from build123d import *

# Parameters (mm, degrees)
SKETCH1_W           = 22.225
SKETCH1_H           = 12.7
BOSS_EXTRUDE1_DEPTH = 50.8
SKETCH2_R           = 1.905
CUT_EXTRUDE1_DEPTH  = 57.884801353
CUT_EXTRUDE2_DEPTH  = 56.811406764
FILLET1_R           = 1.5875
SKETCH6_R           = 2.286
CUT_EXTRUDE3_DEPTH  = 57.884801482


with BuildPart() as part:
    # Sketch1 → Boss-Extrude1 (new body)
    with BuildSketch(Plane(origin=(0, 0, 0), x_dir=(1, 0, 0), z_dir=(0, 1, 0))):
        with Locations((11.1125, 6.35)):
            Rectangle(SKETCH1_W, SKETCH1_H)
    extrude(amount=BOSS_EXTRUDE1_DEPTH)

    # Sketch2 → Cut-Extrude1 (cut, through all)
    with BuildSketch(Plane(origin=(0, 0, -12.7), x_dir=(-1, 0, 0), z_dir=(0, 0, -1))):
        with Locations((-17.4625, 44.45)):
            Circle(SKETCH2_R)
        with Locations((-17.4625, 6.35)):
            Circle(SKETCH2_R)
        with Locations((-4.7625, 44.45)):
            Circle(SKETCH2_R)
        with Locations((-4.7625, 6.35)):
            Circle(SKETCH2_R)
    extrude(amount=-CUT_EXTRUDE1_DEPTH, mode=Mode.SUBTRACT)

    # Sketch3 → Cut-Extrude2 (cut, through all)
    with BuildSketch(Plane(origin=(0, 0, -6.35), x_dir=(-1, 0, 0), z_dir=(0, 0, -1))):
        with BuildLine():
            Line((0, 10.541), (0, 2.159))
            Line((0, 2.159), (-0.79375, 2.159))
            ThreePointArc((-0.79375, 2.159), (-1.786060968, 2.860879553), (-2.286, 3.96875))
            Line((-2.286, 3.96875), (-2.286, 8.73125))
            ThreePointArc((-2.286, 8.73125), (-1.786060968, 9.839120447), (-0.79375, 10.541))
            Line((-0.79375, 10.541), (0, 10.541))
        make_face()
    extrude(amount=-CUT_EXTRUDE2_DEPTH, mode=Mode.SUBTRACT)

    # Sketch5 → Cut-Revolve2 (revolve, cut)
    with BuildSketch(Plane(origin=(0, 0, -6.35), x_dir=(-1, 0, 0), z_dir=(0, 0, -1))):
        with BuildLine():
            Line((0, 6.35), (-2.286, 6.35))
            Line((-2.286, 6.35), (-2.286, 8.73125))
            ThreePointArc((-2.286, 8.73125), (-1.786060968, 9.839120447), (-0.79375, 10.541))
            Line((-0.79375, 10.541), (0, 10.541))
            Line((0, 10.541), (0, 6.35))
        make_face()
    revolve(axis=Axis((2.286, 6.35, -6.35), (-1, 0, 0)), mode=Mode.SUBTRACT)

    # Fillet1
    fillet1_edges = [part.edges().sort_by_distance(p)[0] for p in [
        (0, 30.6705, 0),
        (0, 1.0795, 0),
        (22.225, 25.4, 0),
    ]]
    fillet(fillet1_edges, radius=FILLET1_R)

    # Sketch6 → Cut-Extrude3 (cut, through all)
    with BuildSketch(Plane(origin=(22.225, 0, 0), x_dir=(0, 0, -1), z_dir=(1, 0, 0))):
        with Locations((6.045199993, 31.75)):
            Circle(SKETCH6_R)
    extrude(amount=-CUT_EXTRUDE3_DEPTH, mode=Mode.SUBTRACT)


solid = part.part
Design review of the part built by this model. Coordinates are the model's own, in mm. A direction names the side the tool comes from. Coordinates: 2 decimals unless noted, no trailing zeros. Write each loop counter-clockwise with the first axis right and the second up, starting at its lowest first coordinate (ties: lowest second). Pieces come first, ordered by that corner, then holes. Notation, with made-up numbers: (-12, -14.5) - (0, -14.5) arc R7 ccw to (0, -5.5) - close; hole circle Ø1 at (82, 41). An arc over 180 degrees is marked (long way). Use one line per item in the form item = value.
Q1. Consider section D-D (y = 44.45). Write out the cut boundary in (x, z) (1 decimal).
Taken from the geometry:
outline = (0, -12.7) - (2.9, -12.7) - (2.9, 0) - (1.6, 0) arc R1.6 ccw to (0, -1.6) - close; (6.7, -12.7) - (15.6, -12.7) - (15.6, 0) - (6.7, 0) - close; (19.4, -12.7) - (22.2, -12.7) - (22.2, -1.6) arc R1.6 ccw to (20.6, 0) - (19.4, 0) - close
Q2. Consider section B-B (z = -11.5). Count the separate pieces of the cut face and the enclosed holes in it, plus the area to 3 significant figures.
Taken from the geometry:
separate_pieces = 1
enclosed_holes = 4
area = 1,080 mm^2
Q3. Machinability: for faces 4 (the cylindrical face through (11.268, 34.017, -5.748)), 5 (the cylindrical face through (1.775, 2.848, -3.219)), which of the approach directions +Z, -Z, +X, -X, +Y, -Y give a long, thin tool a straight path to every point of the face, cutting with its end or side? Answer none if there is none.
Taken from the geometry:
face_4 = +X, -X
face_5 = +Z, -X
Q4. Consider section C-C (y = 31.75). Write out the cut boundary in (x, z) (1 decimal), plus the area to 3 significant figures.
Taken from the geometry:
outline = (0, -12.7) - (22.2, -12.7) - (22.2, -8.3) - (0, -8.3) - close; (0, -3.8) - (22.2, -3.8) - (22.2, -1.6) arc R1.6 ccw to (20.6, 0) - (1.6, 0) arc R1.6 ccw to (0, -1.6) - close
area = 180 mm^2
Q5. Consider section A-A (x = 6). Write out the cut boundary in (y, z).
Taken from the geometry:
outline = (0, -12.7) - (4.9, -12.7) - (4.9, 0) - (0, 0) - close; (7.8, -12.7) - (43, -12.7) - (43, 0) - (7.8, 0) - close; (45.9, -12.7) - (50.8, -12.7) - (50.8, 0) - (45.9, 0) - close; hole circle Ø4.57 at (31.75, -6.05)
Q6. The part is to be moulded in two halves that separate along X. For faces 1 (the cylindrical face through (19.366, 44.534, -6.439)), 2 (the flat face through (11, 25, -12.7)), 3 (the cylindrical face through (1.797, 9.826, -3.219)), say which applies: +X half, -X half, draft (parallel to the pull), parting line (faces both ways), or undercut.
Taken from the geometry:
face_1 = undercut
face_2 = draft
face_3 = -X half
Q7. For probe 1 along X at (y, z) = (44.5, -5.75) (3 decimals); probe 2 along Y at (x, z) = (5.75, -4.75); probe 3 along Z at (x, y) = (1.5, 19.5), list the stretches that pass through material, from the lowest coordinate up.
Taken from the geometry:
probe_1 = 0 to 2.858, 6.667 to 15.558, 19.367 to 22.225
probe_2 = 0 to 4.72, 7.98 to 29.87, 33.63 to 42.82, 46.08 to 50.8
probe_3 = -12.7 to 0
Q8. Insertion check: pin 1 Ø1.5 at (x, y) = (18.5, 42) entering from +Z; pin 2 Ø4 at (y, z) = (6, -1.5) entering from -X; pin 3 Ø5 at (y, z) = (7, -3) entering from -X. Each pin has a flat end and moves straight along its axis. Give the tip position at first contact, or say it passes through.
Taken from the geometry:
pin_1 = 0
pin_2 = 2.29
pin_3 = 2.02
